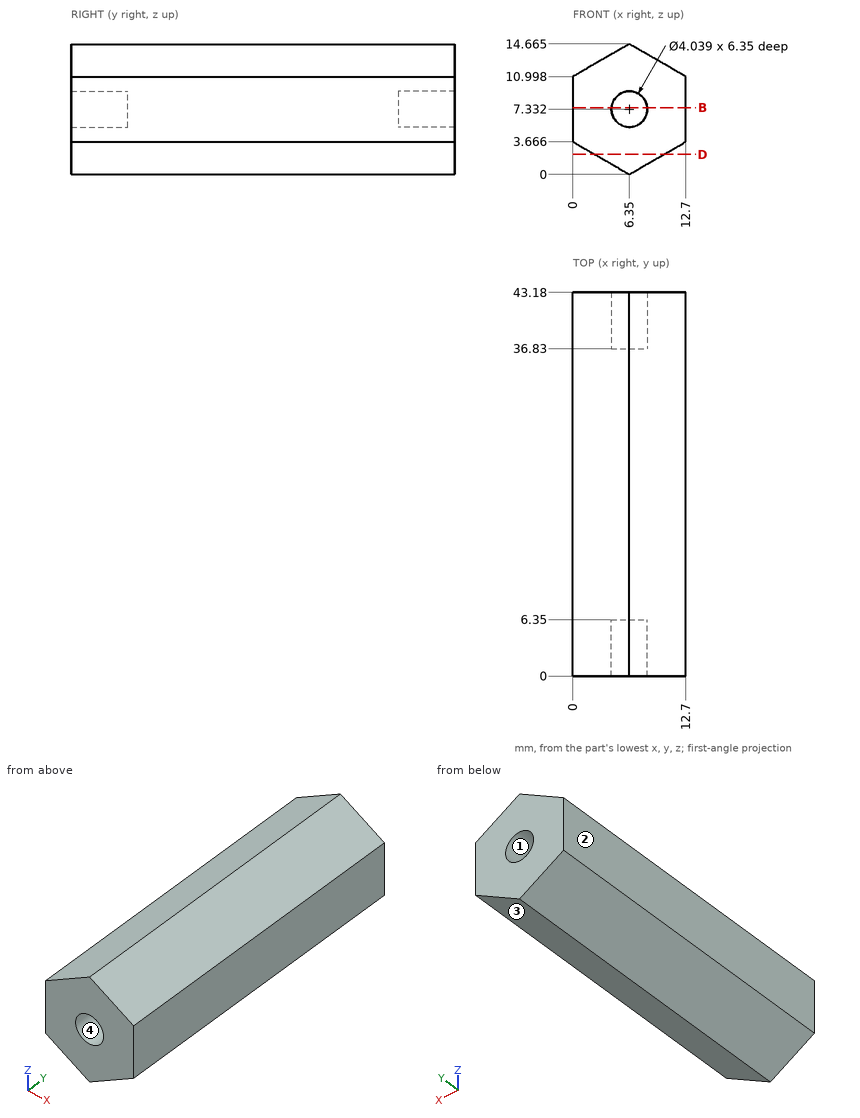
Check sheet for the drawn part. Datum: minimum x, y, z corner. Units: mm. Coordinates: 2 decimals unless noted, no trailing zeros. Loops run counter-clockwise (first coordinate to the right, second up) from the corner with the lowest first, then second, coordinate; pieces in that order, holes last. Notation, with made-up numbers: (23.5, -38.75) -> (72.5, -38.75) arc R20 cw to (72.5, -6.75) -> close; hole circle Ø1 at (19, 36). An arc over 180 degrees is marked (long way). Answer in a Markdown table with one row per item.
1) Draft check along X on the marked faces 1, 2, 3 and 4. Enter one of: released by +X, released by -X, zero draft, split by the parting line, or undercut.
The answers:
| item | result |
|---|---|
| face 1 | undercut |
| face 2 | released by -X |
| face 3 | released by +X |
| face 4 | undercut |
2) Section check D-D (z = 2.25). Record the cut outline in (x, y).
The answers:
| item | result |
|---|---|
| outline | (2.45, 0) -> (10.25, 0) -> (10.25, 43.18) -> (2.45, 43.18) -> close |
3) Section check B-B (z = 7.5). Record the cut outline in (x, y).
The answers:
| item | result |
|---|---|
| outline | (0, 0) -> (4.34, 0) -> (4.34, 6.35) -> (8.36, 6.35) -> (8.36, 0) -> (12.7, 0) -> (12.7, 43.18) -> (8.36, 43.18) -> (8.36, 36.83) -> (4.34, 36.83) -> (4.34, 43.18) -> (0, 43.18) -> close |
4) Scan lines: line 1 along X through (y, z) = (40.5, 7.5); line 2 along Z through (x, y) = (6.5, 38) (1 decimal); line 3 along X through (y, z) = (35.5, 3.5) (1 decimal). Record each from-to range of solid material in increasing order. Write a range as from..to.
The answers:
| item | result |
|---|---|
| line 1 | x = 0..4.34, 8.36..12.7 |
| line 2 | z = 0.1..5.3, 9.3..14.6 |
| line 3 | x = 0.3..12.4 |
5) Depth check by flat-ended pin: P1, Ø1.2, axis at x = 7, z = 8, coming from the -Y side. Enter the tip coordinate at first touch or a pass-through.
The answers:
| item | result |
|---|---|
| P1 | stops at y = 6.35 |
